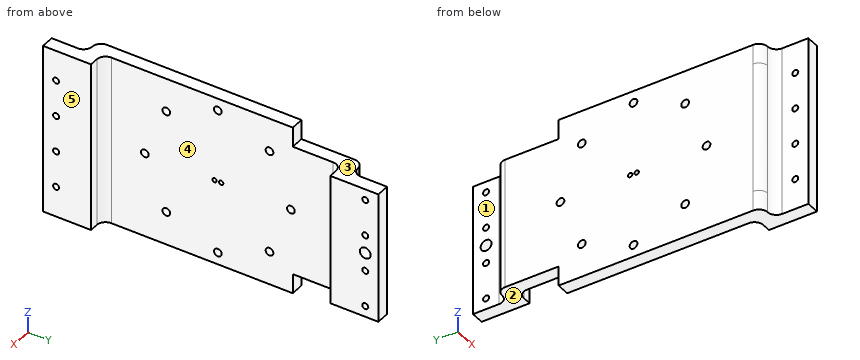
```python
from build123d import *

# Parameters (mm, degrees)
BOSS_EXTRUDE1_DEPTH = 38.1
FILLET1_R           = 5.08
BOSS_EXTRUDE2_DEPTH = 49.53
SKETCH7_R           = 2.25
CUT_EXTRUDE1_DEPTH  = 7.62
SKETCH8_R           = 1.75
CUT_EXTRUDE2_DEPTH  = 7.62
SKETCH10_R          = 3.175
CGTEST1_DEPTH       = 7.62
SKETCH11_R          = 1.27
CUT_EXTRUDE4_DEPTH  = 7.62


with BuildPart() as part:
    # Sketch1 → Boss-Extrude1 (new, symmetric)
    with BuildSketch(Plane.XY):
        Polygon((0, 0), (0, 139.272298857), (10.16, 139.272298857), (10.16, 146.892298857), (10.16, 167.212298857), (2.54, 167.212298857), (2.54, 146.892298857), (-7.62, 146.892298857), (-7.62, 139.272298857), (-7.62, -7.62), (2.54, -7.62), (2.54, -27.94), (10.16, -27.94), (10.16, -7.62), (10.16, 0), align=None)
    extrude(amount=BOSS_EXTRUDE1_DEPTH, both=True)

    # Fillet1
    fillet1_edges = [part.edges().sort_by_distance(p)[0] for p in [
        (0, 0, 0),
        (2.54, -7.62, 0),
        (0, 139.272298857, 0),
        (2.54, 146.892298857, 0),
        (-7.62, 146.892298857, 0),
        (-7.62, -7.62, 0),
    ]]
    fillet(fillet1_edges, radius=FILLET1_R - 0.0001)  # a hair under: the kernel refuses the full size

    # Sketch3 → Boss-Extrude2 (add, symmetric)
    with BuildSketch(Plane(origin=(0, 0, 0), x_dir=(-1, 0, 0), z_dir=(0, 0, -1))):
        with BuildLine():
            Line((0, 110.7), (7.62, 110.7))
            Line((7.62, 110.7), (7.62, -2.54))
            ThreePointArc((7.62, -2.54), (6.132102448, -6.132102448), (2.54, -7.62))
            ThreePointArc((2.54, -7.62), (-1.052102448, -9.107897552), (-2.54, -12.7))
            Line((-2.54, -12.7), (-2.54, -27.94))
            Line((-2.54, -27.94), (-10.16, -27.94))
            Line((-10.16, -27.94), (-10.16, 0))
            Line((-10.16, 0), (-5.08, 0))
            ThreePointArc((-5.08, 0), (-1.487897552, 1.487897552), (0, 5.08))
            Line((0, 5.08), (0, 110.7))
        make_face()
    extrude(amount=BOSS_EXTRUDE2_DEPTH, both=True)

    # Sketch7 → Cut-Extrude1 (cut)
    with BuildSketch(Plane(origin=(0, 0, 0), x_dir=(0, 0, -1), z_dir=(1, 0, 0))):
        with Locations((-42.5, 67.096149428)):
            Circle(SKETCH7_R)
        with Locations((-30.0520382, 97.148187629)):
            Circle(SKETCH7_R)
        with Locations((0, 109.596149428)):
            Circle(SKETCH7_R)
        with Locations((30.0520382, 97.148187629)):
            Circle(SKETCH7_R)
        with Locations((42.5, 67.096149428)):
            Circle(SKETCH7_R)
        with Locations((30.0520382, 37.044111228)):
            Circle(SKETCH7_R)
        with Locations((0, 24.596149428)):
            Circle(SKETCH7_R)
        with Locations((-30.0520382, 37.044111228)):
            Circle(SKETCH7_R)
    extrude(amount=-CUT_EXTRUDE1_DEPTH, mode=Mode.SUBTRACT)

    # Sketch8 → Cut-Extrude2 (cut)
    with BuildSketch(Plane.ZY.offset(-2.54)):
        with Locations(Location((-31.75, 159.592298857, 0), (0, 0, 270))):
            Circle(SKETCH8_R)
        with Locations(Location((-10.583333333, 159.592298857, 0), (0, 0, 270))):
            Circle(SKETCH8_R)
        with Locations(Location((10.583333333, 159.592298857, 0), (0, 0, 270))):
            Circle(SKETCH8_R)
        with Locations(Location((31.75, 159.592298857, 0), (0, 0, 270))):
            Circle(SKETCH8_R)
    cut_extrude2 = extrude(amount=-CUT_EXTRUDE2_DEPTH, mode=Mode.SUBTRACT)

    # Mirror1: Cut-Extrude2 across plane
    add(cut_extrude2.mirror(Plane.ZX.offset(69.636149428)), mode=Mode.SUBTRACT)

    # Sketch10 → CGTest1 (cut)
    with BuildSketch(Plane(origin=(10.16, 0, 0), x_dir=(0, 0, -1), z_dir=(1, 0, 0))):
        with Locations(Location((0, 159.592298857, 0), (0, 0, 90))):
            Circle(SKETCH10_R)
    extrude(amount=-CGTEST1_DEPTH, mode=Mode.SUBTRACT)

    # Sketch11 → Cut-Extrude4 (cut)
    with BuildSketch(Plane.ZY.offset(7.62)):
        with Locations((0, 69.001149428)):
            Circle(SKETCH11_R)
        with Locations((0, 65.191149428)):
            Circle(SKETCH11_R)
    extrude(amount=-CUT_EXTRUDE4_DEPTH, mode=Mode.SUBTRACT)


solid = part.part
```
Part model, mm, in its own coordinate system. Face numbers are marked on the shaded views. A direction names the side the tool comes from. Round coordinates to 2 decimals unless told otherwise and drop trailing zeros. Loops run counter-clockwise (first coordinate to the right, second up) from the corner with the lowest first, then second, coordinate; pieces in that order, holes last. Notation, with made-up numbers: (41.25, 37) -> (76.25, 37) arc R23 ccw to (76.25, 59) -> close; hole circle Ø7 at (56.25, 61.5). An arc over 180 degrees is marked (long way). Use one line per item in the form item = value. Start each with the question number.
Item 1: Band-saw the part on B-B (y = 56). List the corners of the cut face in (x, z).
Item 2: Drop flat-ended pins along their axis: pin 1 Ø8.5 at (x, z) = (-5, 46.5) entering from +Y; pin 2 Ø12 at (y, z) = (58.5, 20) entering from +X; pin 3 Ø3 at (y, z) = (-20.32, 10.58) entering from -X; pin 4 Ø5 at (x, z) = (-4.5, -32.5) entering from +Y. Give the stop position or say it passes through.
Item 3: Two-plate mould, pull along Y, no slides. Class the marked faces 4 and 5: released by +Y, released by -Y, zero draft, split by the parting line, or undercut.
Item 4: Band-saw the part on A-A (z = 42.5). List the corners of the cut face in (x, y), plus the area to 3 significant figures.
Item 5: Drill centre lines: line 1 along Y through (x, z) = (-4.5, -29.5); line 2 along Y through (x, z) = (3.75, -31); line 3 along Y through (x, z) = (-3.5, 0). Where is each one in solid material? Low to high.
Item 6: Tool access for the marked faces 1, 2 and 3: list every direction of +Z, -Z, +X, -X, +Y, -Y with a clear straight run to the whole face (end or side of a thin tool).
Data:
q1.outline = (-7.62, -49.53) -> (0, -49.53) -> (0, 49.53) -> (-7.62, 49.53) -> close
q2.pin_1 = 110.7
q2.pin_2 = 0
q2.pin_3 = through
q2.pin_4 = 146.92
q3.face_4 = undercut
q3.face_5 = zero draft
q4.outline = (-7.62, -2.54) arc R5.08 ccw to (-2.54, -7.62) arc R5.08 cw to (2.54, -12.7) -> (2.54, -27.94) -> (10.16, -27.94) -> (10.16, 0) -> (5.08, 0) arc R5.08 cw to (0, 5.08) -> (0, 64.85) -> (-7.62, 64.85) -> close; (-7.62, 69.35) -> (0, 69.35) -> (0, 110.7) -> (-7.62, 110.7) -> close
q4.area = 1,110 mm^2
q5.line_1 = -7.23 to 34.86, 39.23 to 94.97, 99.33 to 146.5
q5.line_2 = -27.94 to -21.9, -18.74 to 0.18, 139.1 to 158.01, 161.17 to 167.21
q5.line_3 = -7.53 to 22.35, 26.85 to 63.92, 66.46 to 67.73, 70.27 to 107.35, 111.85 to 146.8
q6.face_1 = +Z, -Z, -X, +Y
q6.face_2 = -Z, +X, -X, +Y
q6.face_3 = +Z, +X, -X, +Y
